Can you work these out from the drawing? Everything is in mm from the part's minimum corner. Coordinates: 2 decimals unless noted, no trailing zeros. Loops run counter-clockwise (first coordinate to the right, second up) from the corner with the lowest first, then second, coordinate; pieces in that order, holes last. Notation, with made-up numbers: (24.5, -15) - (34.5, -15) arc R22 ccw to (34.5, 3) - close; hole circle Ø1 at (-30.5, 73.5). An arc over 180 degrees is marked (long way). Use CSV: the item, a comma, the result in double quotes.
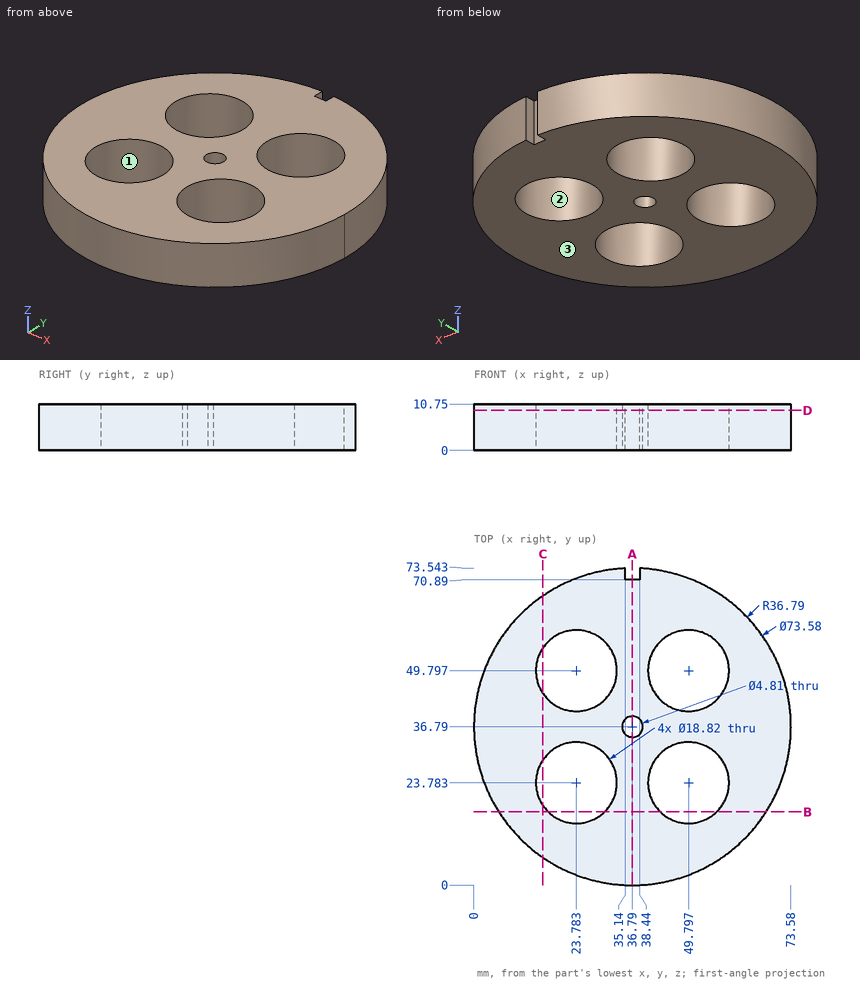
(1) Suppose I cut it at B-B (y = 17). State how many separate pieces and enclosed holes the cut face has, plus the area to 3 significant figures.
Computed:
separate pieces,"3"
enclosed holes,"0"
area,"386 mm²"
(2) Please list where these lines run through material, in increasing order: line 1 (X direction, y = 16.5, z = 1.5) (1 decimal); line 2 (X direction, y = 54, z = 5); line 3 (Y direction, x = 47.5, z = 3.75).
Computed:
line 1,"x = 6.1 to 17.8, 29.7 to 43.8, 55.8 to 67.5"
line 2,"x = 4.27 to 15.36, 32.2 to 41.38, 58.22 to 69.31"
line 3,"y = 1.59 to 14.66, 32.91 to 40.67, 58.92 to 71.99"
(3) Will these pins go through, and if not, where does the flat tip stop? pin 1 (21.5 mm diameter, centred on x = 49.8, y = 23.78, fed in from +Z); pin 2 (3 mm diameter, centred on y = 32, z = 8, fed in from +X); pin 3 (1.3 mm diameter, centred on y = 71.5, z = 6.5, fed in from -X); pin 4 (4 mm diameter, centred on y = 58, z = 5, fed in from +X).
Computed:
pin 1,"stops at z = 10.75"
pin 2,"stops at x = 73.43"
pin 3,"stops at x = 22.88"
pin 4,"stops at x = 68.17"
(4) Suppose I cut it at D-D (z = 9.25). Write out the boundary of the cut face in (x, y) (1 decimal).
Computed:
outline,"(35.1, 70.9) - (35.1, 73.5) arc R36.8 ccw (long way) to (38.4, 73.5) - (38.4, 70.9) - close; hole circle Ø18.8 at (23.8, 23.8); hole circle Ø18.8 at (23.8, 49.8); hole circle Ø4.8 at (36.8, 36.8); hole circle Ø18.8 at (49.8, 23.8); hole circle Ø18.8 at (49.8, 49.8)"
(5) Suppose I cut it at A-A (x = 36.79). Write out the boundary of the cut face in (y, z) (3 decimals), plus the area to 3 significant figures.
Computed:
outline,"(0, 0) - (34.385, 0) - (34.385, 10.75) - (0, 10.75) - close; (39.195, 0) - (70.89, 0) - (70.89, 10.75) - (39.195, 10.75) - close"
area,"710 mm²"
(6) Suppose I cut it at C-C (x = 16). Write out the boundary of the cut face in (y, z), plus the area to 3 significant figures.
Computed:
outline,"(6.44, 0) - (18.49, 0) - (18.49, 10.75) - (6.44, 10.75) - close; (29.07, 0) - (44.51, 0) - (44.51, 10.75) - (29.07, 10.75) - close; (55.09, 0) - (67.14, 0) - (67.14, 10.75) - (55.09, 10.75) - close"
area,"425 mm²"
(7) Thinking about a two-plate mould opening in X: for the marked faces 1, 2 and 3, which applies, +X half, -X half, draft (parallel to the pull), parting line (faces both ways), or undercut?
Computed:
face 1,"undercut"
face 2,"undercut"
face 3,"draft"
